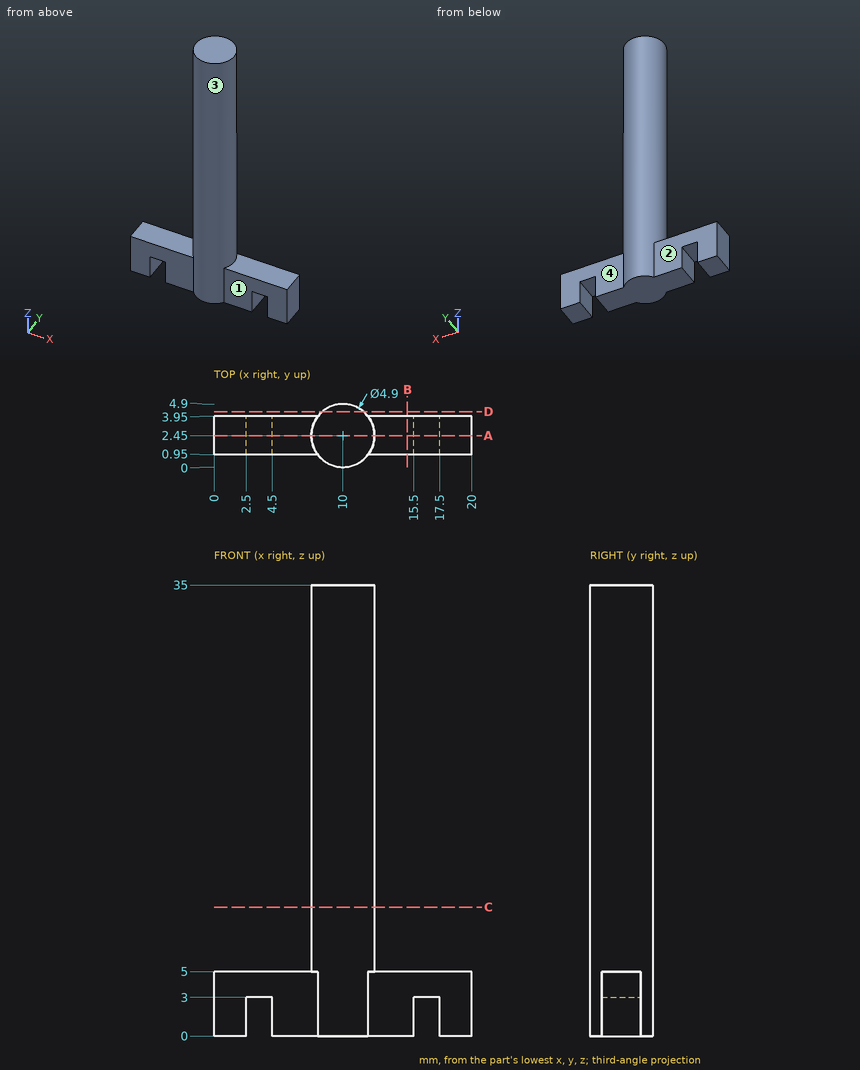
Study the drawing (mm; zero at the part's minimum x, y, z) and answer. A direction names the side the tool comes from. Give positions to 0.01 mm unless a question says otherwise; leave off trailing zeros. Write each loop counter-clockwise with the first axis right and the second up, starting at its lowest first coordinate (ties: lowest second). Pieces come first, ordered by that corner, then holes. Notation, with made-up numbers: (35.25, 54.25) - (57.25, 54.25) arc R10 cw to (57.25, 65.25) - close; hole circle Ø5 at (-11.75, 18.5). An arc over 180 degrees is marked (long way). Use CSV: the item, a comma, the result in double quotes. Start each with the question number.
(1) Find section C-C (z = 10). Give the vertices of the cut face in (x, y), plus the area to 3 significant figures.
(2) Consider line 1 along X through (y, z) = (2, 2.5); line 2 along Z through (x, y) = (5.5, 3.5); line 3 along Z through (x, y) = (17.25, 2.8). Determine where each line is inside the solid, lowest interval first.
(3) Find section B-B (x = 15). Give the vertices of the cut face in (y, z).
(4) For the marked faces 1, 2, 3 and 4, determine the directions among +Z, -Z, +X, -X, +Y, -Y from which every point of the face is accessible in a straight line to the end or side of a thin tool.
(5) Find section D-D (y = 4.3). Give the vertices of the cut face in (x, z), plus the area to 3 significant figures.
(6) Find section A-A (y = 2.45). Give the vertices of the cut face in (x, z), plus the area to 3 significant figures.
(7) Given P1, Ø5.5, axis at x = 18, z = 3.5, coming from the +Y side; P2, Ø4, axis at x = 13, z = 4, coming from the -Y side; P3, Ø5.5, axis at x = 17, z = 3.5, coming from the -Y side, each flat-ended and moving along its own axis, determine where each tip first touches the part or whether it passes through.
Findings below:
1,outline,"circle Ø4.9 at (10, 2.45)"
1,area,"18.9 mm2"
2,line 1,"0 to 2.5, 4.5 to 15.5, 17.5 to 20"
2,line 2,"0 to 5"
2,line 3,"3 to 5"
3,outline,"(0.95, 0) - (3.95, 0) - (3.95, 5) - (0.95, 5) - close"
4,face 1,"+Z, -Z, +X, -Y"
4,face 2,"+Z, -Z, -X, +Y"
4,face 3,"+Z"
4,face 4,"+Z, -Z, +X, +Y"
5,outline,"(8.39, 0) - (11.61, 0) - (11.61, 35) - (8.39, 35) - close"
5,area,"112 mm2"
6,outline,"(0, 0) - (2.5, 0) - (2.5, 3) - (4.5, 3) - (4.5, 0) - (15.5, 0) - (15.5, 3) - (17.5, 3) - (17.5, 0) - (20, 0) - (20, 5) - (12.45, 5) - (12.45, 35) - (7.55, 35) - (7.55, 5) - (0, 5) - close"
6,area,"235 mm2"
7,P1,"y = 3.95"
7,P2,"y = 0.21"
7,P3,"y = 0.95"
